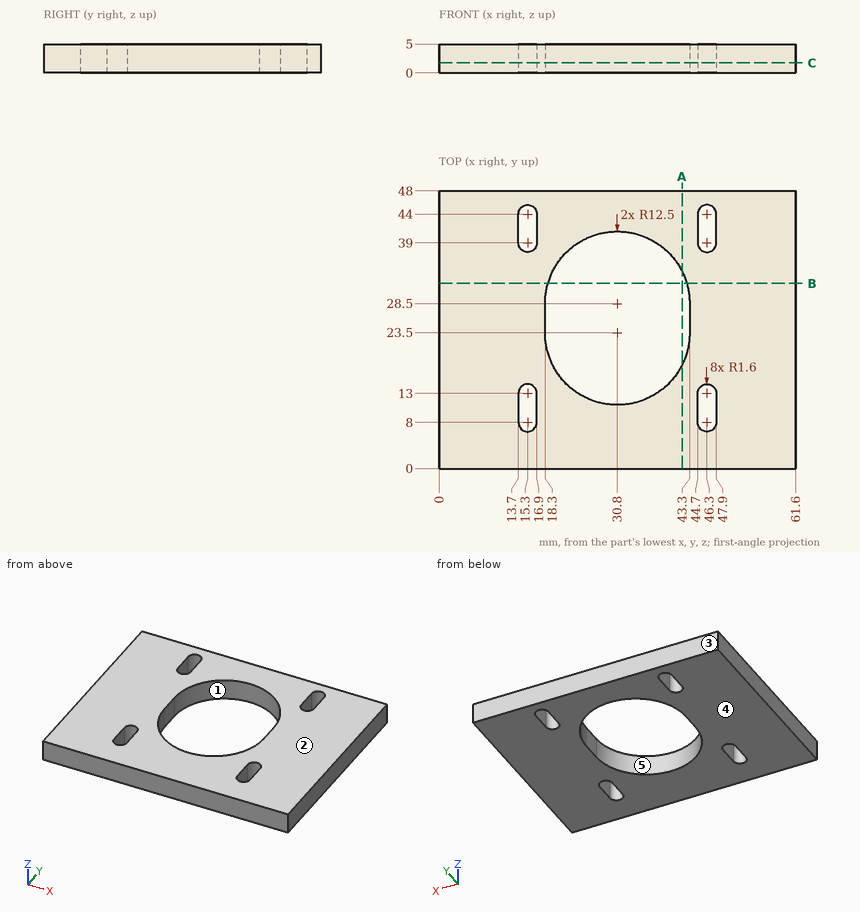
Source: three-view drawing plus pictorial views. Frame: mm from the lowest corner of the part. A direction names the side the tool comes from. Give positions to 0.01 mm unless a question says otherwise; leave off trailing zeros. Order: outer loops, then holes, each group sorted by start corner. A loop starts at its lowest first (then second) coordinate and runs counter-clockwise, first axis right, second up. Notation, with made-up numbers: (-20, -10) - (-8, -10) arc R22 ccw to (-8, -3) - close; hole circle Ø8 at (75, -27.75). An arc over 180 degrees is marked (long way). Put each result on its own line as item: value.
Item 1: Access query for the marked faces 4 and 5. Directions: +Z, -Z, +X, -X, +Y, -Y. A direction counts if a zero-diameter tool reaches every point of the face in a straight line with its end or side. Return the directions, or none.
Found:
face 4: -Z, +X, -X, +Y, -Y
face 5: +Z, -Z
Item 2: Section query B-B, the plane y = 32. Return loops of the section in (x, z), then the cut area to 3 significant figures.
Found:
outline: (0, 0) - (18.8, 0) - (18.8, 5) - (0, 5) - close; (42.8, 0) - (61.6, 0) - (61.6, 5) - (42.8, 5) - close
area: 188 mm^2
Item 3: Draft query along Y for the marked faces 1, 2 and 3. Return one class per face: +Y half, -Y half, draft (parallel to the pull), parting line (faces both ways), or undercut.
Found:
face 1: undercut
face 2: draft
face 3: +Y half
Item 4: Section query A-A, the plane x = 42. Return loops of the section in (y, z), then the cut area to 3 significant figures.
Found:
outline: (0, 0) - (17.95, 0) - (17.95, 5) - (0, 5) - close; (34.05, 0) - (48, 0) - (48, 5) - (34.05, 5) - close
area: 159 mm^2
Item 5: Section query C-C, the plane z = 1.75. Return loops of the section in (x, y), then the cut area to 3 significant figures.
Found:
outline: (0, 0) - (61.6, 0) - (61.6, 48) - (0, 48) - close; hole (13.7, 8) arc R1.6 ccw to (16.9, 8) - (16.9, 13) arc R1.6 ccw to (13.7, 13) - close; hole (13.7, 39) arc R1.6 ccw to (16.9, 39) - (16.9, 44) arc R1.6 ccw to (13.7, 44) - close; hole (18.3, 23.5) arc R12.5 ccw to (43.3, 23.5) - (43.3, 28.5) arc R12.5 ccw to (18.3, 28.5) - close; hole (44.7, 8) arc R1.6 ccw to (47.9, 8) - (47.9, 13) arc R1.6 ccw to (44.7, 13) - close; hole (44.7, 39) arc R1.6 ccw to (47.9, 39) - (47.9, 44) arc R1.6 ccw to (44.7, 44) - close
area: 2,240 mm^2
Item 6: Ray query, L1, parallel to X at y = 8.5, z = 0.35; L2, parallel to X at y = 29, z = 4.05; L3, parallel to X at y = 39, z = 0.95. Return the intervals inside material, ascending. Write a range as from..to.
Found:
L1: x = 0..13.7, 16.9..44.7, 47.9..61.6
L2: x = 0..18.31, 43.29..61.6
L3: x = 0..13.7, 16.9..24.02, 37.58..44.7, 47.9..61.6
